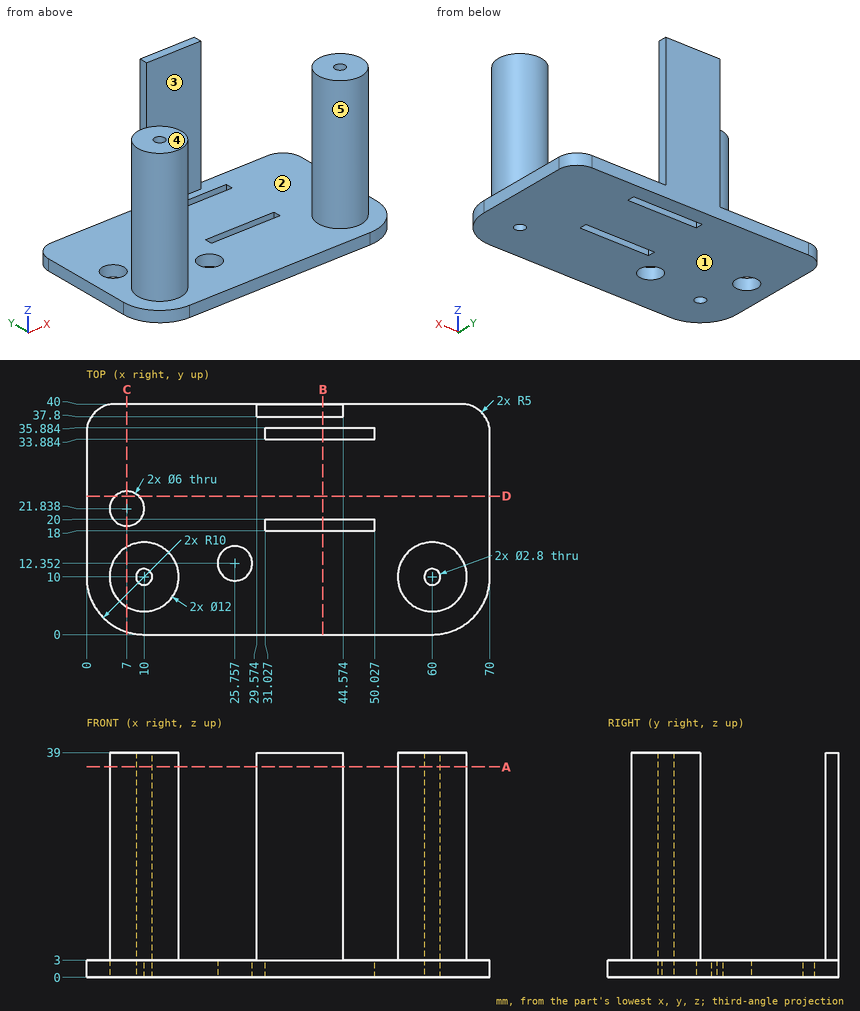
Can you work these out from the drawing? Everything is in mm from the part's minimum corner. A direction names the side the tool comes from. Round coordinates to 2 decimals unless told otherwise and drop trailing zeros. Order: outer loops, then holes, each group sorted by start corner. A loop starts at its lowest first (then second) coordinate and runs counter-clockwise, first axis right, second up. Notation, with made-up numbers: M 42,69 L 54,69 A23 cw 54,94 Z; hole C 71.5,12.25 d8. An arc over 180 degrees is marked long. Answer as CSV lines item,"result".
Item 1: Imagine slicing it at B-B on x = 41. List the corners of the cut face in (y, z) for me (1 decimal).
From the geometry:
outline,"M 0,0 L 18,0 L 18,3 L 0,3 Z; M 20,0 L 33.9,0 L 33.9,3 L 20,3 Z; M 35.9,0 L 40,0 L 40,39 L 37.8,39 L 37.8,3 L 35.9,3 Z"
Item 2: Imagine slicing it at C-C on x = 7. List the corners of the cut face in (y, z) for me.
From the geometry:
outline,"M 0.46,0 L 18.84,0 L 18.84,3 L 15.2,3 L 15.2,39 L 4.8,39 L 4.8,3 L 0.46,3 Z; M 24.84,0 L 40,0 L 40,3 L 24.84,3 Z"
Item 3: Imagine slicing it at D-D on y = 24. List the corners of the cut face in (x, z) for me.
From the geometry:
outline,"M 0,0 L 4.92,0 L 4.92,3 L 0,3 Z; M 9.08,0 L 70,0 L 70,3 L 9.08,3 Z"
Item 4: Which directions (+Z, -Z, +X, -X, +Y, -Y) give clear straight access to the entire face, cutting with the end or side of a thin tool? Please do the marked faces 3, 4 and 5.
From the geometry:
face 3,"+Z, +X, -X, -Y"
face 4,"+Z, +X, -X, +Y, -Y"
face 5,"+Z"
Item 5: We'd pull the mould along X, two halves only. Please class the marked faces 1 and 2: +X half, -X half, draft (parallel to the pull), parting line (faces both ways), or undercut.
From the geometry:
face 1,"draft"
face 2,"undercut"
Item 6: Please list where these lines run through material, in increasing order: L1, parallel to Y at x = 60, z = 26; L2, parallel to Z at x = 43, y = 36; L3, parallel to Y at x = 32, z = 9. Write a range as [from, to].
From the geometry:
L1,"[4, 8.6], [11.4, 16]"
L2,"[0, 3]"
L3,"[37.8, 40]"
Item 7: For pin 1 (2 mm diameter, centred on x = 7, z = 9, fed in from -Y); pin 2 (4 mm diameter, centred on y = 28.5, z = 5.5, fed in from +X); pin 3 (2.5 mm diameter, centred on y = 39.5, z = 18.5, fed in from -X); pin 4 (1.5 mm diameter, centred on x = 40.5, z = 1, fed in from -Y), each with a flat end and sliding along its axis, tell me the tip position at first contact or that it passes through.
From the geometry:
pin 1,"y = 4.34"
pin 2,"through"
pin 3,"x = 29.57"
pin 4,"y = 0"
Item 8: Imagine slicing it at A-A on z = 36.5. List the corners of the cut face in (x, y) for me.
From the geometry:
outline,"C 10,10 d12; M 29.57,37.8 L 44.57,37.8 L 44.57,40 L 29.57,40 Z; C 60,10 d12; hole C 10,10 d2.8; hole C 60,10 d2.8"
